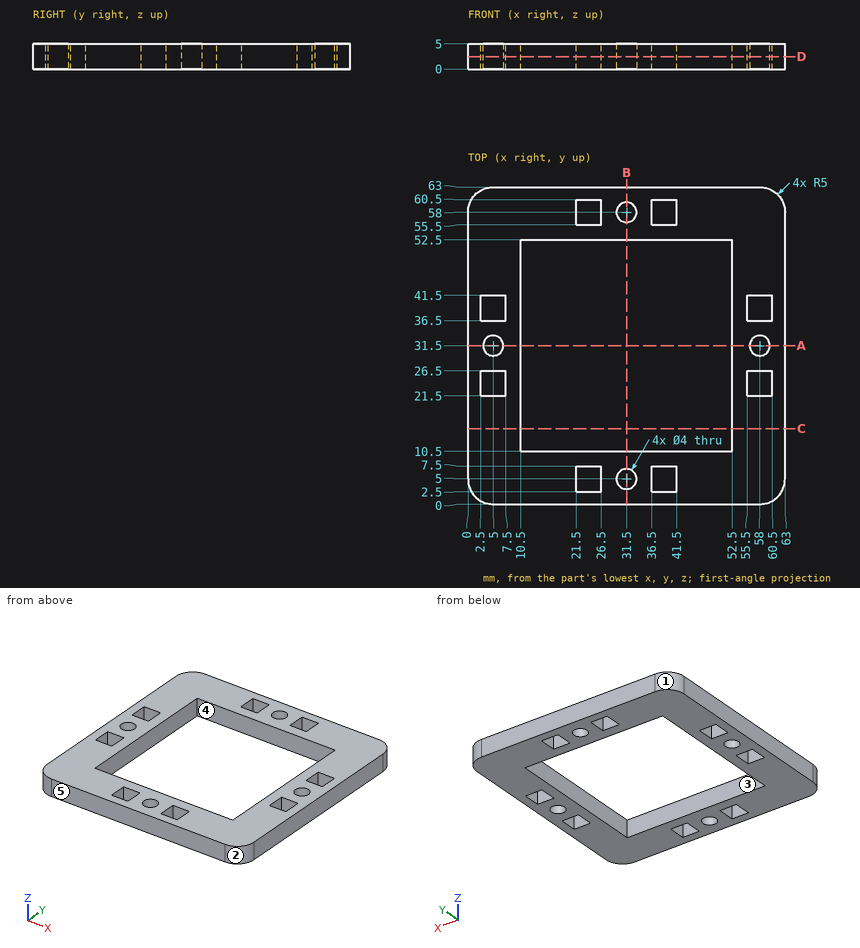
The drawing under review shows one solid part. Ordinate dimensions are in mm from its lowest x, y, z. A direction names the side the tool comes from. Round coordinates to 2 decimals unless told otherwise and drop trailing zeros. Loops run counter-clockwise (first coordinate to the right, second up) from the corner with the lowest first, then second, coordinate; pieces in that order, holes last. Notation, with made-up numbers: (79.25, -19) - (103.25, -19) arc R6 ccw to (103.25, -8) - close; hole circle Ø2 at (18, 85.5). An arc over 180 degrees is marked (long way). One line per question, with ' | ' between items.
1. Draft analysis for pull direction X (two halves, no side actions). For the marked faces 1, 2 and 3, state which applies: released by +X, released by -X, zero draft, split by the parting line, or undercut.
Results are:
face 1: released by -X | face 2: released by +X | face 3: undercut
2. For the marked faces 4 and 5, list the 3-axis set-ups (+Z, -Z, +X, -X, +Y, -Y) from which the entire face can be reached by the end or side of a thin tool; tool diameter is ignored.
Results are:
face 4: +Z, -Z | face 5: +Z, -Z, +X, -X, -Y
3. For L1, parallel to Y at x = 5, z = 3.5; L2, parallel to Y at x = 25, z = 4.3, list the stretches that pass through material, from the lowest coordinate up. Write a range as [from, to].
Results are:
L1: y = [0, 21.5], [26.5, 29.5], [33.5, 36.5], [41.5, 63] | L2: y = [0, 2.5], [7.5, 10.5], [52.5, 55.5], [60.5, 63]
4. We need section D-D, the plane z = 2.5. State how many separate pieces and enclosed holes the cut face has, and give its area (3 significant figures).
Results are:
separate pieces: 1 | enclosed holes: 13 | area: 1,930 mm²
5. We need section A-A, the plane y = 31.5. State the section outline as (x, z) points, and give its area (3 significant figures).
Results are:
outline: (0, 0) - (3, 0) - (3, 5) - (0, 5) - close; (7, 0) - (10.5, 0) - (10.5, 5) - (7, 5) - close; (52.5, 0) - (56, 0) - (56, 5) - (52.5, 5) - close; (60, 0) - (63, 0) - (63, 5) - (60, 5) - close | area: 65.0 mm²
6. Clearance check with a flat-ended pin moving along its axis: P1, Ø12, axis at x = 16, y = 17.5, coming from the -Z side. State where the tip first meets the part, or that it passes through.
Results are:
P1: stops at z = 0
7. We need section C-C, the plane y = 15. State the section outline as (x, z) points.
Results are:
outline: (0, 0) - (10.5, 0) - (10.5, 5) - (0, 5) - close; (52.5, 0) - (63, 0) - (63, 5) - (52.5, 5) - close
